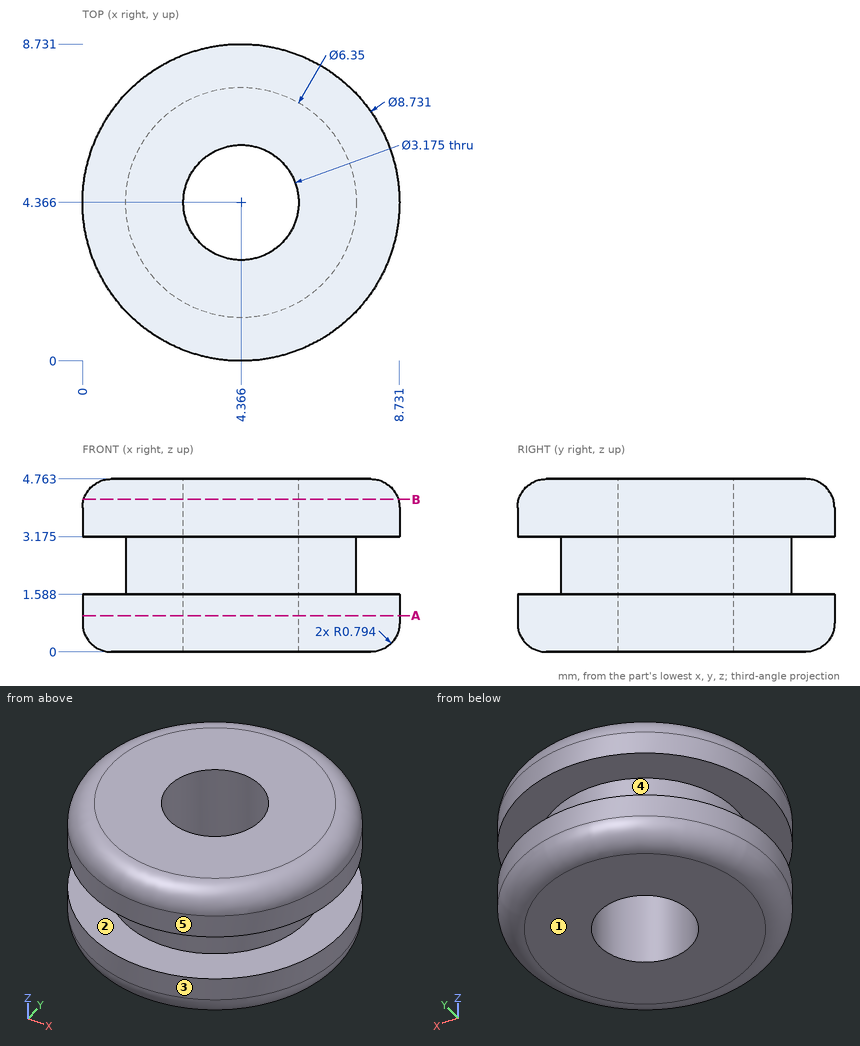
Could you check a few things on this drawing? It's one solid part, dimensions in mm from its lowest x, y, z. A direction names the side the tool comes from. Coordinates: 2 decimals unless noted, no trailing zeros. Write each loop counter-clockwise with the first axis right and the second up, starting at its lowest first coordinate (ties: lowest second). Pieces come first, ordered by that corner, then holes. Notation, with made-up numbers: (4.25, -10) - (9.25, -10) arc R28 ccw to (9.25, 21) - close; hole circle Ø1 at (40, -10). An arc over 180 degrees is marked (long way). Write item = value, one per line.
1) For the marked faces 4 and 5, which set-ups out of +Z, -Z, +X, -X, +Y, -Y let a thin tool reach every point of the face, with its end or its side?
Result set:
face_4 = none
face_5 = +Z, -Z
2) Suppose I cut it at A-A on z = 1. Please give me the cut outline in (x, y) (1 decimal).
Result set:
outline = circle Ø8.7 at (4.4, 4.4); hole circle Ø3.2 at (4.4, 4.4)
3) We'd pull the mould along Z, two halves only. Please class the marked faces 1, 2 and 3: +Z half, -Z half, draft (parallel to the pull), parting line (faces both ways), or undercut.
Result set:
face_1 = -Z half
face_2 = undercut
face_3 = draft
4) Please list where these lines run through material, in increasing order: line 1 (Z direction, x = 3.75, y = 7.75) (1 decimal); line 2 (Y direction, x = 3.5, z = 3.65) (1 decimal); line 3 (Y direction, x = 6.5, z = 4.5) (1 decimal). Write a range as [from, to].
Result set:
line_1 = [0, 1.6], [3.2, 4.8]
line_2 = [0.1, 3], [5.7, 8.6]
line_3 = [0.8, 7.9]
5) Will these pins go through, and if not, where does the flat tip stop? pin 1 Ø1 at (y, z) = (6.5, 1) entering from -X; pin 2 Ø1 at (y, z) = (5.5, 2) entering from -X.
Result set:
pin_1 = 0.32
pin_2 = 0.08
